Part model, mm, in its own coordinate system. A direction names the side the tool comes from. Round coordinates to 2 decimals unless told otherwise and drop trailing zeros. Order: outer loops, then holes, each group sorted by start corner. A loop starts at its lowest first (then second) coordinate and runs counter-clockwise, first axis right, second up. Notation, with made-up numbers: (-12.5, 64.5) - (-1.5, 64.5) arc R16 ccw to (-1.5, 71.5) - close; hole circle Ø4 at (63.25, 62). An arc over 180 degrees is marked (long way). Answer as a JSON object with one key per item and string values.
```python
from build123d import *

# Parameters (mm, degrees)
F0_W     = 224.0026
F0_H     = 72.9996
F1_DEPTH = 12.7
F2_W     = 178.2826
F2_H     = 47.5996
F2_W_2   = 173.2026
F2_H_2   = 22.1996
F3_DEPTH = 25.4
F4_W     = 8.89
F4_H     = 11.43
F5_DEPTH = 508
F6_W     = 8.89
F6_H     = 11.43
F7_DEPTH = 508
F8_R     = 2.54
F9_DEPTH = 508


with BuildPart() as f1:
    # F0 (on Top) → F1 (new body)
    with BuildSketch(Plane.XY):
        Rectangle(F0_W, F0_H)
    extrude(amount=F1_DEPTH)

    # F2 (on face) → F3 (cut)
    with BuildSketch(Plane.XY.offset(12.7)):
        Rectangle(F2_W, F2_H)
        Rectangle(F2_W_2, F2_H_2, mode=Mode.SUBTRACT)
        Rectangle(F2_W_2, F2_H_2)
    extrude(amount=-F3_DEPTH, mode=Mode.SUBTRACT)

    # F4 (on face) → F5 (cut)
    with BuildSketch(Plane.YZ.offset(112.0013)):
        with Locations((-32.0548, 5.715)):
            Rectangle(F4_W, F4_H)
    extrude(amount=-F5_DEPTH, mode=Mode.SUBTRACT)

    # F6 (on face) → F7 (cut)
    with BuildSketch(Plane.YZ.offset(112.0013)):
        with Locations((32.0548, 5.715)):
            Rectangle(F6_W, F6_H)
    extrude(amount=-F7_DEPTH, mode=Mode.SUBTRACT)

    # F8 (on face) → F9 (cut)
    with BuildSketch(Plane.YZ.offset(112.0013)):
        with Locations((0, 6.35)):
            Circle(F8_R)
    extrude(amount=-F9_DEPTH, mode=Mode.SUBTRACT)


solid = f1.part
```
Item 1: Cut at A-A (z = 6.35). Write the cut outline in (x, y), plus the area to 3 significant figures.
Taken from the geometry:
{"outline": "(-112, -27.61) - (112, -27.61) - (112, -2.54) - (89.14, -2.54) - (89.14, -23.8) - (-89.14, -23.8) - (-89.14, -2.54) - (-112, -2.54) - close; (-112, 2.54) - (-89.14, 2.54) - (-89.14, 23.8) - (89.14, 23.8) - (89.14, 2.54) - (112, 2.54) - (112, 27.61) - (-112, 27.61) - close", "area": "3,650 mm2"}
Item 2: Probe L1, parallel to X at y = -4, z = 5; L2, parallel to Y at x = -27.5, z = 11.25; L3, parallel to Z at x = -104, y = 0. List the from-to ranges inside material, lowest first. Write a range as from..to.
Taken from the geometry:
{"L1": "-112..-89.14, 89.14..112", "L2": "-27.61..-23.8, 23.8..27.61", "L3": "0..3.81, 8.89..12.7"}
Item 3: Cut at D-D (y = -13). Write the cut outline in (x, z), plus the area to 3 significant figures.
Taken from the geometry:
{"outline": "(-112, 0) - (-89.14, 0) - (-89.14, 12.7) - (-112, 12.7) - close; (89.14, 0) - (112, 0) - (112, 12.7) - (89.14, 12.7) - close", "area": "581 mm2"}
Item 4: Cut at C-C (x = 31). Write the cut outline in (y, z).
Taken from the geometry:
{"outline": "(-36.5, 11.43) - (-27.61, 11.43) - (-27.61, 0) - (-23.8, 0) - (-23.8, 12.7) - (-36.5, 12.7) - close; (23.8, 0) - (27.61, 0) - (27.61, 11.43) - (36.5, 11.43) - (36.5, 12.7) - (23.8, 12.7) - close"}
Item 5: Cut at B-B (y = 0). Write the cut outline in (x, z), plus the area to 3 significant figures.
Taken from the geometry:
{"outline": "(-112, 0) - (-89.14, 0) - (-89.14, 3.81) - (-112, 3.81) - close; (-112, 8.89) - (-89.14, 8.89) - (-89.14, 12.7) - (-112, 12.7) - close; (89.14, 0) - (112, 0) - (112, 3.81) - (89.14, 3.81) - close; (89.14, 8.89) - (112, 8.89) - (112, 12.7) - (89.14, 12.7) - close", "area": "348 mm2"}
Item 6: Drop flat-ended pins along their axis: P1, Ø10, axis at x = 34, y = 31.5, coming from the -Z side; P2, Ø2.5, axis at x = -28.5, y = -30.5, coming from the -Z side; P3, Ø4.5, axis at y = 0, z = 6.35, coming from the -X side; P4, Ø3.5, axis at x = -4, z = 4, coming from the +Y side. Give the stop position or say it passes through.
Taken from the geometry:
{"P1": "z = 0", "P2": "z = 11.43", "P3": "through", "P4": "y = 27.61"}
Item 7: Tool access for faces 5 (the flat face through (-89.141, -0.3, 3.6)), 6 (the flat face through (2, -27.61, 6)), 7 (the flat face through (2, 32, 11.43)), 8 (the flat face through (112.001, -1, 9)): list every direction of +Z, -Z, +X, -X, +Y, -Y with a clear straight run to the whole face (end or side of a thin tool).
Taken from the geometry:
{"face 5": "+Z, -Z", "face 6": "-Z, +X, -X, -Y", "face 7": "-Z, +X, -X, +Y", "face 8": "+Z, -Z, +X, +Y, -Y"}
Item 8: Two-plate mould, pull along X, no slides. Class faces 1 (the flat face through (-1, 23.8, 6)), 2 (the flat face through (-112.001, -1, 9)), 3 (the flat face through (89.141, -0.3, 3.6)), 4 (the flat face through (-2, -24, 0)): pulls with the +X half, pulls with the -X half, needs draft (parallel to the pull), parting line crosses it, or undercut.
Taken from the geometry:
{"face 1": "undercut", "face 2": "pulls with the -X half", "face 3": "undercut", "face 4": "needs draft"}
